Autodesk Inventor part; units mm, degrees
ref_plane "YZ Plane" through (0, 0, 0) normal (1, 0, 0) x (0, 1, 0)
ref_plane "XZ Plane" through (0, 0, 0) normal (0, 1, 0) x (-1, 0, 0)
ref_plane "XY Plane" through (0, 0, 0) normal (0, 0, 1) x (1, 0, 0)
sketch "Esquisse1" plane through (0, 0, 0) normal (0, 0, 1) x (1, 0, 0)
  circle A0 centre (0, 0) radius 7.9
  circle A1 centre (0, 0) radius 4
  dimension "d0" = 15.8
  dimension "d1" = 8
extrude "Extrusion1" add sketch "Esquisse1" along normal blind 65
sketch "Esquisse2" plane through (0, 0, 0) normal (0, 1, 0) x (-1, 0, 0)
  line L0 (7.9, 65) -> (-7.9, 65)
  line L1 (0, 65) -> (0, 60)
  line L2 (0, 0) -> (0, 5)
  dimension "d4" = 5
  dimension "d5" = 5
hole "Perçage1" at (0, 0, 60) at (0, 0, 5) direction (0, -1, 0) diameter 4 end through all both
properties part number "tube vers roue libre"
Can you work these out from the model? Positions are in its coordinate system, mm. Round coordinates to 2 decimals unless told otherwise and drop trailing zeros. Loops run counter-clockwise (first coordinate to the right, second up) from the corner with the lowest first, then second, coordinate; pieces in that order, holes last. Notation, with made-up numbers: (50, 23) -> (79, 23) arc R21 cw to (79, 37) -> close; hole circle Ø3 at (5.25, 68.5). An arc over 180 degrees is marked (long way). Answer in a Markdown table with one row per item.
Item 1: Suppose I cut it at D-D, the plane z = 36.5. List the corners of the cut face in (x, y) for me.
Answer block:
| item | result |
|---|---|
| outline | circle Ø15.8 at (0, 0); hole circle Ø8 at (0, 0) |
Item 2: If I drill on probe 1 along Z at (x, y) = (0, 6.05); probe 2 along Y at (x, z) = (0, 10.5); probe 3 along Z at (x, y) = (-1.5, 5), over which ranges is the centre line in solid material (lowest first)?
Answer block:
| item | result |
|---|---|
| probe 1 | 0 to 3, 7 to 58, 62 to 65 |
| probe 2 | -7.9 to -4, 4 to 7.9 |
| probe 3 | 0 to 3.68, 6.32 to 58.68, 61.32 to 65 |
Item 3: We'd pull the mould along X, two halves only. Please class faces 1 (the cylindrical face through (1.846, 3.549, 32.045)), 2 (the flat face through (-4, 2, 0)), 3 (the cylindrical face through (7.535, -2.373, 32.045)): released by +X, released by -X, zero draft, split by the parting line, or undercut.
Answer block:
| item | result |
|---|---|
| face 1 | undercut |
| face 2 | zero draft |
| face 3 | split by the parting line |
Item 4: Suppose I cut it at C-C, the plane z = 60. List the corners of the cut face in (x, y) for me.
Answer block:
| item | result |
|---|---|
| outline | (-2, -7.64) -> (-2, -3.46) arc R4 cw to (-2, 3.46) -> (-2, 7.64) arc R7.9 ccw to start; (2, -7.64) arc R7.9 ccw to (2, 7.64) -> (2, 3.46) arc R4 cw to (2, -3.46) -> close |
Item 5: Suppose I cut it at B-B, the plane x = 0. List the corners of the cut face in (y, z) for me, plus the area to 3 significant figures.
Answer block:
| item | result |
|---|---|
| outline | (-7.9, 0) -> (-4, 0) -> (-4, 3) -> (-7.9, 3) -> close; (-7.9, 7) -> (-4, 7) -> (-4, 58) -> (-7.9, 58) -> close; (-7.9, 62) -> (-4, 62) -> (-4, 65) -> (-7.9, 65) -> close; (4, 0) -> (7.9, 0) -> (7.9, 3) -> (4, 3) -> close; (4, 7) -> (7.9, 7) -> (7.9, 58) -> (4, 58) -> close; (4, 62) -> (7.9, 62) -> (7.9, 65) -> (4, 65) -> close |
| area | 445 mm² |
Item 6: Suppose I cut it at A-A, the plane y = 0. List the corners of the cut face in (x, z) for me, plus the area to 3 significant figures.
Answer block:
| item | result |
|---|---|
| outline | (-7.9, 0) -> (-4, 0) -> (-4, 65) -> (-7.9, 65) -> close; (4, 0) -> (7.9, 0) -> (7.9, 65) -> (4, 65) -> close |
| area | 507 mm² |
Item 7: Will these pins go through, and if not, where does the flat tip stop? P1, Ø5, axis at y = -3.5, z = 7, coming from the +X side; P2, Ø1.5, axis at y = 1.5, z = 47, coming from the +X side; P3, Ø2.5, axis at x = 0, z = 60, coming from the +Y side; P4, Ø4, axis at x = 2.5, z = 54.5, coming from the -Y side.
Answer block:
| item | result |
|---|---|
| P1 | x = 7.84 |
| P2 | x = 7.86 |
| P3 | through |
| P4 | y = -7.88 |
